The listing builds one solid part. Answer for the finished solid, in the listing's coordinates (mm). A direction names the side the tool comes from. Give positions to 0.01 mm unless a question says otherwise; leave off trailing zeros. Write each loop counter-clockwise with the first axis right and the second up, starting at its lowest first coordinate (ties: lowest second). Pieces come first, ordered by that corner, then holes. Notation, with made-up numbers: (21, -11) -> (74, -11) arc R27 ccw to (74, 23) -> close; hole circle Ø2 at (79.25, 30.25). An arc over 180 degrees is marked (long way). One line per question, with ' | ' between items.
from build123d import *

# Parameters (mm, degrees)
SKETCH1_R               = 10.5
BOSS_EXTRUDE1_DEPTH     = 82
BOSS_EXTRUDE2_START     = 3
SKETCH1_3_R             = 10.5
BOSS_EXTRUDE2_DEPTH     = 3
CUT_EXTRUDE1_DEPTH      = 115.585426104
CUT_EXTRUDE1_DEPTH_BACK = 115.585426104
SKETCH2_W               = 66
SKETCH2_H               = 93.23561667
FILLET1_R               = 5
FILLET2_R               = 2


with BuildPart() as part:
    # Sketch1 → Boss-Extrude1 (new body)
    # profile 1 of 3: a face of its own
    with BuildSketch(Plane.XY):
        with BuildLine():
            Line((4, 14.456832295), (-4, 14.456832295))
            ThreePointArc((-4, 14.456832295), (-9.082951062, -11.937336386), (15, 0))
            ThreePointArc((15, 0), (11.937336386, 9.082951062), (4, 14.456832295))
        make_face()
        Circle(SKETCH1_R, mode=Mode.SUBTRACT)
    # profile 2 of 3: a face of its own
    with BuildSketch(Plane.XY):
        with BuildLine():
            Line((-4, 74.456832295), (-4, 14.456832295))
            ThreePointArc((-4, 14.456832295), (0, 15), (4, 14.456832295))
            Line((4, 14.456832295), (4, 74.456832295))
            Line((4, 74.456832295), (-4, 74.456832295))
        make_face()
    # profile 3 of 3: a face of its own
    with BuildSketch(Plane.XY):
        with BuildLine():
            ThreePointArc((4, 14.456832295), (0, 15), (-4, 14.456832295))
            Line((-4, 14.456832295), (4, 14.456832295))
        make_face()
    extrude(amount=-BOSS_EXTRUDE1_DEPTH)

    # Sketch1<3> → Boss-Extrude2 (add)
    # profile 1 of 2: a face of its own
    with BuildSketch(Plane.XY.offset(BOSS_EXTRUDE2_START)):
        with BuildLine():
            Line((4, 14.456832295), (-4, 14.456832295))
            ThreePointArc((-4, 14.456832295), (-9.082951062, -11.937336386), (15, 0))
            ThreePointArc((15, 0), (11.937336386, 9.082951062), (4, 14.456832295))
        make_face()
        Circle(SKETCH1_3_R, mode=Mode.SUBTRACT)
    # profile 2 of 2: a face of its own
    with BuildSketch(Plane.XY.offset(BOSS_EXTRUDE2_START)):
        with BuildLine():
            ThreePointArc((4, 14.456832295), (0, 15), (-4, 14.456832295))
            Line((-4, 14.456832295), (4, 14.456832295))
        make_face()
    boss_extrude2 = extrude(amount=-BOSS_EXTRUDE2_DEPTH)

    # Mirror1: Boss-Extrude2 across plane
    add(boss_extrude2.mirror(Plane.XY.offset(-41)))

    # Sketch2 → Cut-Extrude1 (cut, two sides: drawn at the far end of the back side and taken through both)
    with BuildSketch(Plane.ZY.offset(4).offset(-CUT_EXTRUDE1_DEPTH_BACK)):
        with Locations((-41, 19.83902396)):
            Rectangle(SKETCH2_W, SKETCH2_H)
    extrude(amount=CUT_EXTRUDE1_DEPTH + CUT_EXTRUDE1_DEPTH_BACK, mode=Mode.SUBTRACT)

    # Fillet1
    fillet1_edges = [part.edges().sort_by_distance(p)[0] for p in [
        (0, 74.456832295, -82),
        (0, 66.456832295, -8),
        (0, 66.456832295, -74),
        (0, 74.456832295, 0),
    ]]
    fillet(fillet1_edges, radius=FILLET1_R)

    # Fillet2
    fillet2_edges = [part.edges().sort_by_distance(p)[0] for p in [
        (-10.5, 0, 3),
        (-4, -14.456832295, 3),
        (-4, -14.456832295, -85),
        (-10.5, 0, -85),
    ]]
    fillet(fillet2_edges, radius=FILLET2_R)


solid = part.part
Item 1: Find section B-B (z = -6.5). Write down the section's boundary in (x, y).
Answers below:
outline: (-4, 14.46) arc R15 ccw (long way) to (4, 14.46) -> (4, 74.46) -> (-4, 74.46) -> close; hole circle Ø21 at (0, 0)
Item 2: Find section A-A (y = 54.5). Write down the section's boundary in (x, z).
Answers below:
outline: (-4, -82) -> (4, -82) -> (4, -74) -> (-4, -74) -> close; (-4, -8) -> (4, -8) -> (4, 0) -> (-4, 0) -> close
Item 3: Find section C-C (x = 0). Count the separate pieces of the cut face and the enclosed holes in it, then the cut area to 3 significant figures.
Answers below:
separate pieces: 3 | enclosed holes: 0 | area: 1,670 mm²
Item 4: Consider line 1 (Z direction, x = -3, y = 34); line 2 (Y direction, x = 0, z = -77); line 3 (Y direction, x = 0, z = -4.25). Determine where each line is inside the solid, lowest interval first. Write a range as [from, to].
Answers below:
line 1: [-82, -74], [-8, 0] | line 2: [-15, -10.5], [10.5, 74.46] | line 3: [-15, -10.5], [10.5, 74.4]
Item 5: Find section D-D (z = -18.5). Write down the section's boundary in (x, y).
Answers below:
outline: (-4, 66.46) -> (4, 66.46) -> (4, 74.46) -> (-4, 74.46) -> close
Item 6: A tool of negligible diameter and unlimited length cuts with its end or side. For faces 4 (the face through (0, 42, 0)), 5 (the face through (4, 67, -44)), 6 (the face through (0, 23, -74)), 7 (the face through (1.78, 12.53, -85)), from which of +Z, -Z, +X, -X, +Y, -Y can it reach the whole face along a straight path? Write none if from no direction.
Answers below:
face 4: +Z, +X, -X, +Y | face 5: +Z, -Z, +X, +Y | face 6: +X, -X, -Y | face 7: -Z, +X, -X, +Y, -Y
Item 7: Determine the mould class of faces 1 (the face through (0, 74.457, -40)), 2 (the face through (-4, 67, -41)), 3 (the face through (10, 3.2, -3.4)) for opening direction X: pulls with the +X half, pulls with the -X half, needs draft (parallel to the pull), parting line crosses it, or undercut.
Answers below:
face 1: needs draft | face 2: pulls with the -X half | face 3: undercut
Item 8: Flat-ended cylindrical pins translate along their axes: pin 1 (9 mm diameter, centred on x = 1, z = -50, fed in from -Y); pin 2 (9 mm diameter, centred on x = -1, y = 30.5, fed in from -Z); pin 3 (10 mm diameter, centred on x = 9.5, z = -6.5, fed in from +Y). Find the tip coordinate at first contact, or state that the pin passes through.
Answers below:
pin 1: y = 66.46 | pin 2: z = -82 | pin 3: y = 14.31
